Verification items for the finished model (mm, model axes). A direction names the side the tool comes from. Coordinates: 2 decimals unless noted, no trailing zeros. Loops run counter-clockwise (first coordinate to the right, second up) from the corner with the lowest first, then second, coordinate; pieces in that order, holes last. Notation, with made-up numbers: (84, 82.5) - (96, 82.5) arc R18 ccw to (96, 87.5) - close; hole circle Ø1 at (50, 26.25). An arc over 180 degrees is marked (long way). Answer as CSV lines item,"result". Start each with the question number.
1. Set-up check for faces 4 (the flat face through (-9.824, -36.663, 1.014)), 5 (the cylindrical face through (-2.504, -11.275, 28.829)): record each of +Z, -Z, +X, -X, +Y, -Y from which the full face is reachable in a straight line by a thin tool's end or side.
2. Cross-section at D-D (x = -37.5). Enter the section's corners in (y, z), plus the area to 3 significant figures.
3. Cross-section at C-C (z = 8.5). Enter the section's corners in (x, y).
4. Cross-section at A-A (x = 0). Enter the section's corners in (y, z), plus the area to 3 significant figures.
5. Material ranges on line 1 (Y direction, x = 15, z = 1.5); line 2 (Y direction, x = 0, z = 3.9); line 3 (Z direction, x = -52, y = -33), recorded low to high. Write a range as [from, to].
6. Release check for a two-part mould opening along X. For faces 1 (the flat face through (0, 12, 52)), 2 (the flat face through (-9, 5, 5)), 3 (the cylindrical face through (-10.316, -7.91, 26.65)) record: pulls with the +X half, pulls with the -X half, needs draft (parallel to the pull), parting line crosses it, or undercut.
7. Cross-section at B-B (y = -33). Enter the section's corners in (x, z), plus the area to 3 significant figures.
8. Gauge pin test, flat ends, axial feed: P1, Ø5, axis at x = 13.5, y = 34, coming from the +Z side; P2, Ø10, axis at x = -11.5, y = 2, coming from the -Z side; P3, Ø11.5, axis at x = -4.5, y = 1.5, coming from the +Z side; P4, Ø6, axis at x = 9.5, z = 40.5, coming from the -Y side. Record the tip position at first contact, or that the pin passes through.
```python
from build123d import *

# Parameters (mm, degrees)
SKETCH1_R           = 62.5
SKETCH1_R_2         = 1.5
BOSS_EXTRUDE1_DEPTH = 2
SKETCH2_R           = 13
BOSS_EXTRUDE2_DEPTH = 50
SKETCH6_R           = 11.55
CUT_EXTRUDE7_DEPTH  = 47
SKETCH7_R           = 10
CUT_EXTRUDE8_DEPTH  = 101.107442281
CUT_EXTRUDE9_DEPTH  = 102.550480058


with BuildPart() as part:
    # Sketch1 → Boss-Extrude1 (new body)
    with BuildSketch(Plane.XY):
        Circle(SKETCH1_R)
        with Locations((-57.5, 0)):
            Circle(SKETCH1_R_2, mode=Mode.SUBTRACT)
        with Locations((0, 57.5)):
            Circle(SKETCH1_R_2, mode=Mode.SUBTRACT)
        with Locations((57.5, 0)):
            Circle(SKETCH1_R_2, mode=Mode.SUBTRACT)
        with Locations((0, -57.5)):
            Circle(SKETCH1_R_2, mode=Mode.SUBTRACT)
        with Locations((-15, 0)):
            Circle(SKETCH1_R_2, mode=Mode.SUBTRACT)
        with Locations(Location((15, 0, 0), (0, 0, 180))):
            Circle(SKETCH1_R_2, mode=Mode.SUBTRACT)
    extrude(amount=BOSS_EXTRUDE1_DEPTH)

    # Sketch2 → Boss-Extrude2 (add)
    with BuildSketch(Plane.XY.offset(2)):
        Circle(SKETCH2_R)
    extrude(amount=BOSS_EXTRUDE2_DEPTH)

    # Sketch6 → Cut-Extrude7 (cut)
    with BuildSketch(Plane.XY.offset(52)):
        Circle(SKETCH6_R)
    extrude(amount=-CUT_EXTRUDE7_DEPTH, mode=Mode.SUBTRACT)

    # Sketch7 → Cut-Extrude8 (cut, through all)
    with BuildSketch(Plane.XY.offset(5)):
        Circle(SKETCH7_R)
    extrude(amount=-CUT_EXTRUDE8_DEPTH, mode=Mode.SUBTRACT)

    # Sector (Cut Extrude) → Cut-Extrude9 (cut, through all)
    with BuildSketch(Plane.XY.offset(2)):
        with BuildLine():
            Line((22.216294005, -5.952838037), (50.71110588, -13.587999868))
            ThreePointArc((50.71110588, -13.587999868), (37.123106012, -37.123106012), (13.587999868, -50.71110588))
            Line((13.587999868, -50.71110588), (5.952838037, -22.216294005))
            ThreePointArc((5.952838037, -22.216294005), (16.263455967, -16.263455967), (22.216294005, -5.952838037))
        make_face()
        with BuildLine():
            Line((-22.216294005, -5.952838037), (-50.71110588, -13.587999868))
            ThreePointArc((-50.71110588, -13.587999868), (-37.123106012, -37.123106012), (-13.587999868, -50.71110588))
            Line((-13.587999868, -50.71110588), (-5.952838037, -22.216294005))
            ThreePointArc((-5.952838037, -22.216294005), (-16.263455967, -16.263455967), (-22.216294005, -5.952838037))
        make_face()
        with BuildLine():
            Line((-5.952838037, 22.216294005), (-13.587999868, 50.71110588))
            ThreePointArc((-13.587999868, 50.71110588), (-37.123106012, 37.123106012), (-50.71110588, 13.587999868))
            Line((-50.71110588, 13.587999868), (-22.216294005, 5.952838037))
            ThreePointArc((-22.216294005, 5.952838037), (-16.263455967, 16.263455967), (-5.952838037, 22.216294005))
        make_face()
        with BuildLine():
            Line((22.216294005, 5.952838037), (50.71110588, 13.587999868))
            ThreePointArc((50.71110588, 13.587999868), (37.123106012, 37.123106012), (13.587999868, 50.71110588))
            Line((13.587999868, 50.71110588), (5.952838037, 22.216294005))
            ThreePointArc((5.952838037, 22.216294005), (16.263455967, 16.263455967), (22.216294005, 5.952838037))
        make_face()
    extrude(amount=-CUT_EXTRUDE9_DEPTH, mode=Mode.SUBTRACT)


solid = part.part
```
Values follow:
1,face 4,"+Z, -Z"
1,face 5,"+Z"
2,outline,"(-50, 0) - (-36.74, 0) - (-36.74, 2) - (-50, 2) - close; (-10.05, 0) - (10.05, 0) - (10.05, 2) - (-10.05, 2) - close; (36.74, 0) - (50, 0) - (50, 2) - (36.74, 2) - close"
2,area,"93.2 mm²"
3,outline,"circle Ø26 at (0, 0); hole circle Ø23.1 at (0, 0)"
4,outline,"(-62.5, 0) - (-59, 0) - (-59, 2) - (-62.5, 2) - close; (-56, 0) - (-10, 0) - (-10, 5) - (-11.55, 5) - (-11.55, 52) - (-13, 52) - (-13, 2) - (-56, 2) - close; (10, 0) - (56, 0) - (56, 2) - (13, 2) - (13, 52) - (11.55, 52) - (11.55, 5) - (10, 5) - close; (59, 0) - (62.5, 0) - (62.5, 2) - (59, 2) - close"
4,area,"352 mm²"
5,line 1,"y = [-60.67, -50.31], [-17.44, -1.5], [1.5, 17.44], [50.31, 60.67]"
5,line 2,"y = [-13, -10], [10, 13]"
5,line 3,"z = [0, 2]"
6,face 1,"needs draft"
6,face 2,"undercut"
6,face 3,"parting line crosses it"
7,outline,"(-53.08, 0) - (-40.83, 0) - (-40.83, 2) - (-53.08, 2) - close; (-8.84, 0) - (8.84, 0) - (8.84, 2) - (-8.84, 2) - close; (40.83, 0) - (53.08, 0) - (53.08, 2) - (40.83, 2) - close"
7,area,"84.4 mm²"
8,P1,"passes through"
8,P2,"stops at z = 0"
8,P3,"stops at z = 5"
8,P4,"stops at y = -11.26"
